```python
from build123d import *

# Parameters (mm, degrees)
EXTRUDE_1_DEPTH          = 2
EXTRUDE_2_DEPTH          = 4
CUT_EXTRUDE_1_DEPTH      = 115.638809515
CUT_EXTRUDE_1_DEPTH_BACK = 115.638809515
CUT_EXTRUDE_2_DEPTH      = 115.638809515
CUT_EXTRUDE_2_DEPTH_BACK = 115.638809515
SKETCH_5_R               = 1
SKETCH_6_W               = 23
SKETCH_6_H               = 3
EXTRUDE_3_DEPTH          = 14


with BuildPart() as part:
    # 草图1 → 凸台-拉伸1 (new, symmetric)
    with BuildSketch(Plane(origin=(0, 0, 0), x_dir=(1, 0, 0), z_dir=(0, 1, 0))):
        with BuildLine():
            Line((-11.5, -10.5), (17.5, -10.5))
            Line((17.5, -10.5), (17.5, 10.5))
            Line((17.5, 10.5), (-11.5, 10.5))
            ThreePointArc((-11.5, 10.5), (-19.5, 0), (-11.5, -10.5))
        make_face()
        Polygon((11.5, -6.5), (-11.5, -6.5), (-11.5, -3), (-12.5, -3), (-12.5, 3), (-11.5, 3), (-11.5, 6.5), (11.5, 6.5), align=None, mode=Mode.SUBTRACT)
    extrude(amount=EXTRUDE_1_DEPTH, both=True)

    # 草图2 → 凸台-拉伸2 (add)
    with BuildSketch(Plane(origin=(0, 2, 0), x_dir=(1, 0, 0), z_dir=(0, 1, 0))):
        with BuildLine():
            Line((17.5, -5.5), (17.5, -10.5))
            ThreePointArc((17.5, -10.5), (59.440835798, -4.44595009), (101.5, -9.614309047))
            ThreePointArc((101.5, -9.614309047), (111.034090536, -14.463041261), (109.336734694, -3.902356171))
            ThreePointArc((109.336734694, -3.902356171), (63.979602253, 6.877540604), (17.5, 10.5))
            Line((17.5, 10.5), (17.5, 6.5))
            ThreePointArc((17.5, 6.5), (47.689236459, 4.99679808), (77.5, 0))
            ThreePointArc((77.5, 0), (47.280596762, -0.356510126), (17.5, -5.5))
        make_face()
    extrude(amount=-EXTRUDE_2_DEPTH)

    # 草图4 → 切除-拉伸1 (cut, two sides: drawn at the far end of the back side and taken through both)
    with BuildSketch(Plane.XZ.offset(2).offset(-CUT_EXTRUDE_1_DEPTH_BACK)):
        with BuildLine():
            Line((102.276706609, 12.566800564), (105.378679656, 11.735629391))
            Line((105.378679656, 11.735629391), (104.547508484, 14.837602438))
            ThreePointArc((104.547508484, 14.837602438), (103.257359313, 13.856949735), (102.276706609, 12.566800564))
        make_face()
        with BuildLine():
            Line((110.452491516, 14.837602438), (109.621320344, 11.735629391))
            Line((109.621320344, 11.735629391), (112.723293391, 12.566800564))
            ThreePointArc((112.723293391, 12.566800564), (111.742640687, 13.856949735), (110.452491516, 14.837602438))
        make_face()
        with BuildLine():
            Line((112.723293391, 6.661817531), (109.621320344, 7.492988704))
            Line((109.621320344, 7.492988704), (110.452491516, 4.391015657))
            ThreePointArc((110.452491516, 4.391015657), (111.742640687, 5.37166836), (112.723293391, 6.661817531))
        make_face()
    extrude(amount=CUT_EXTRUDE_1_DEPTH + CUT_EXTRUDE_1_DEPTH_BACK, mode=Mode.SUBTRACT)

    # 草图5 → 切除-拉伸2 (cut, two sides: drawn at the far end of the back side and taken through both)
    with BuildSketch(Plane.XZ.offset(2).offset(-CUT_EXTRUDE_2_DEPTH_BACK)):
        with Locations(Location((14.5, 0, 0), (0, 0, 270))):
            Circle(SKETCH_5_R)
        with Locations(Location((-14.5, 0, 0), (0, 0, 270))):
            Circle(SKETCH_5_R)
    extrude(amount=CUT_EXTRUDE_2_DEPTH + CUT_EXTRUDE_2_DEPTH_BACK, mode=Mode.SUBTRACT)

    # 草图6 → 凸台-拉伸3 (add)
    with BuildSketch(Plane(origin=(0, 2, 0), x_dir=(1, 0, 0), z_dir=(0, 1, 0))):
        with Locations((0, -8)):
            Rectangle(SKETCH_6_W, SKETCH_6_H)
    extrude_3 = extrude(amount=EXTRUDE_3_DEPTH)

    # 镜向1: 凸台-拉伸3 across plane
    add(extrude_3.mirror(Plane.XY))


solid = part.part
```
Geometry check sheet. Reference: the model listing, model coordinates, mm. A direction names the side the tool comes from. Round coordinates to 2 decimals unless told otherwise and drop trailing zeros. Loops run counter-clockwise (first coordinate to the right, second up) from the corner with the lowest first, then second, coordinate; pieces in that order, holes last. Notation, with made-up numbers: (71, 14) - (93, 14) arc R24 ccw to (93, 44) - close; hole circle Ø10 at (-15, -40). An arc over 180 degrees is marked (long way). Use a Markdown table: item, result.
Q1. Cross-section at B-B on x = 0. Record the cut outline in (y, z), plus the area to 3 significant figures.
Solutions:
| item | result |
|---|---|
| outline | (-2, -10.5) - (2, -10.5) - (2, -9.5) - (16, -9.5) - (16, -6.5) - (-2, -6.5) - close; (-2, 6.5) - (16, 6.5) - (16, 9.5) - (2, 9.5) - (2, 10.5) - (-2, 10.5) - close |
| area | 116 mm2 |
Q2. Cross-section at C-C on z = -4.5. Record the cut outline in (x, y), plus the area to 3 significant figures.
Solutions:
| item | result |
|---|---|
| outline | (-18.53, -2) - (-11.5, -2) - (-11.5, 2) - (-18.53, 2) - close; (11.5, -2) - (17.5, -2) - (17.5, 2) - (11.5, 2) - close; (51.95, -2) - (77.2, -2) - (77.2, 2) - (51.95, 2) - close |
| area | 153 mm2 |
Q3. Cross-section at A-A on y = 7.5. Record the cut outline in (x, z), plus the area to 3 significant figures.
Solutions:
| item | result |
|---|---|
| outline | (-11.5, -9.5) - (11.5, -9.5) - (11.5, -6.5) - (-11.5, -6.5) - close; (-11.5, 6.5) - (11.5, 6.5) - (11.5, 9.5) - (-11.5, 9.5) - close |
| area | 138 mm2 |
Q4. Go/stop test with flat-tipped pins: P1, Ø3.5, axis at y = 11, z = -7.5, coming from the +X side; P2, Ø3.5, axis at y = 7, z = 8, coming from the -X side; P3, Ø4, axis at x = 5, y = 5.5, coming from the +Z side; P4, Ø1.8, axis at x = -14.5, z = 0, coming from the -Y side. Record where each tip stops, or that it passes through.
Solutions:
| item | result |
|---|---|
| P1 | stops at x = 11.5 |
| P2 | stops at x = -11.5 |
| P3 | stops at z = 9.5 |
| P4 | passes through |
Q5. Access from +Z, -Z, +X, -X, +Y, -Y to the whole of each face (thin tool, end or side, straight path). Record for faces 4 (the flat face through (0, 16, 8)), 5 (the cylindrical face through (101.69, 0.03, 11.12)), 6 (the flat face through (46, -2, 2)), 7 (the flat face through (-11.5, 9, -8)), 8 (the flat face through (0, 7, -6.5)).
Solutions:
| item | result |
|---|---|
| face 4 | +Z, -Z, +X, -X, +Y |
| face 5 | +Z, +Y, -Y |
| face 6 | +Z, -Z, +X, -X, -Y |
| face 7 | +Z, -Z, -X, +Y |
| face 8 | +Y, -Y |
Q6. Material ranges on line 1 (Z direction, x = -8.5, y = 0.5); line 2 (Z direction, x = 14.5, y = -0.75); line 3 (Y direction, x = 35.5, z = 4.75), recorded low to high.
Solutions:
| item | result |
|---|---|
| line 1 | z = -10.5 to -6.5, 6.5 to 10.5 |
| line 2 | z = -10.5 to -1, 1 to 10.5 |
| line 3 | y = -2 to 2 |
Q7. Draft check along X on faces 1 (the flat face through (0, 16, -8)), 2 (the cylindrical face through (-19.5, 0, -0.2)), 3 (the flat face through (104.97, 0.03, 13.26)). Enter one of: released by +X, released by -X, zero draft, split by the parting line, or undercut.
Solutions:
| item | result |
|---|---|
| face 1 | zero draft |
| face 2 | released by -X |
| face 3 | undercut |
Q8. Cross-section at D-D on x = 54. Record the cut outline in (y, z).
Solutions:
| item | result |
|---|---|
| outline | (-2, -8.27) - (2, -8.27) - (2, -4.23) - (-2, -4.23) - close; (-2, -0.14) - (2, -0.14) - (2, 4.6) - (-2, 4.6) - close |
